from build123d import *

# Parameters (mm, degrees)
SKETCH_1_W            = 80
SKETCH_1_H            = 35
SKETCH_1_R            = 1.5
EXTRUDE_1_DEPTH       = 1.5
EXTRUDE_START         = 7
EXTRUDE_2_OUTLINE_W   = 71
EXTRUDE_2_OUTLINE_H   = 6
EXTRUDE_2_OUTLINE_H_2 = 2
EXTRUDE_2_DEPTH       = 22.5
EXTRUDE_2_2_OUTLINE_W = 44.5
EXTRUDE_2_2_OUTLINE_H = 10
EXTRUDE_2_2_DEPTH     = 3.5


# Read off the part's stored shape, not the designer's step: Бобышка-Вытянуть2
with BuildPart() as part:
    # Эскиз1 (on Top Plane) → Бобышка-Вытянуть1 (new body)
    with BuildSketch(Plane(origin=(0, 0, 0), x_dir=(1, 0, 0), z_dir=(0, 1, 0))):
        with Locations((40, -17.5)):
            Rectangle(SKETCH_1_W, SKETCH_1_H)
        with Locations(Location((2.5, -2, 0), (0, 0, 270))):
            Circle(SKETCH_1_R, mode=Mode.SUBTRACT)
        with Locations(Location((77.5, -2, 0), (0, 0, 90))):
            Circle(SKETCH_1_R, mode=Mode.SUBTRACT)
        with Locations(Location((77.5, -33, 0), (0, 0, 270))):
            Circle(SKETCH_1_R, mode=Mode.SUBTRACT)
        with Locations(Location((2.5, -33, 0), (0, 0, 90))):
            Circle(SKETCH_1_R, mode=Mode.SUBTRACT)
    extrude(amount=EXTRUDE_1_DEPTH)

    # Бобышка-Вытянуть2 outline → Бобышка-Вытянуть2 (add)
    with BuildSketch(Plane.XY.offset(EXTRUDE_START)):
        with Locations((40, 4.5)):
            Rectangle(EXTRUDE_2_OUTLINE_W, EXTRUDE_2_OUTLINE_H)
        with Locations((40, -1)):
            Rectangle(EXTRUDE_2_OUTLINE_W, EXTRUDE_2_OUTLINE_H_2)
    extrude(amount=EXTRUDE_2_DEPTH)

    # Extrude 2 2 outline → Extrude 2 2 (add)
    with BuildSketch(Plane.XY):
        with Locations((27.75, -5)):
            Rectangle(EXTRUDE_2_2_OUTLINE_W, EXTRUDE_2_2_OUTLINE_H)
    extrude(amount=EXTRUDE_2_2_DEPTH)


solid = part.part
Verification items for the finished model (mm, model axes). A direction names the side the tool comes from. Give positions to 0.01 mm unless a question says otherwise; leave off trailing zeros. Order: outer loops, then holes, each group sorted by start corner. A loop starts at its lowest first (then second) coordinate and runs counter-clockwise, first axis right, second up. Notation, with made-up numbers: (72.25, 20.25) -> (108.25, 20.25) arc R20 ccw to (108.25, 26.25) -> close; hole circle Ø6 at (9, -31.5). An arc over 180 degrees is marked (long way). Answer as CSV lines item,"result".
Q1. Sectioned sample at D-D on z = 15. Record the cut outline in (x, y), plus the area to 3 significant figures.
Solutions:
outline,"(0, 0) -> (4.5, 0) -> (4.5, -2) -> (75.5, -2) -> (75.5, 0) -> (80, 0) -> (80, 1.5) -> (75.5, 1.5) -> (75.5, 7.5) -> (4.5, 7.5) -> (4.5, 1.5) -> (0, 1.5) -> close"
area,"688 mm²"
Q2. Sectioned sample at C-C on x = 77.5. Record the cut outline in (y, z), plus the area to 3 significant figures.
Solutions:
outline,"(0, 0) -> (1.5, 0) -> (1.5, 0.5) -> (0, 0.5) -> close; (0, 3.5) -> (1.5, 3.5) -> (1.5, 31.5) -> (0, 31.5) -> close; (0, 34.5) -> (1.5, 34.5) -> (1.5, 35) -> (0, 35) -> close"
area,"43.5 mm²"
Q3. Sectioned sample at A-A on y = -1. Record the cut outline in (x, z), plus the area to 3 significant figures.
Solutions:
outline,"(4.5, 7) -> (75.5, 7) -> (75.5, 29.5) -> (4.5, 29.5) -> close; (5.5, 0) -> (50, 0) -> (50, 3.5) -> (5.5, 3.5) -> close"
area,"1,750 mm²"
Q4. Depth check by flat-ended pin: pin 1 (12 mm diameter, centred on x = 30, z = 15.5, fed in from -Y); pin 2 (3 mm diameter, centred on y = 3.5, z = 17, fed in from +X); pin 3 (1.8 mm diameter, centred on x = 2.5, z = 33, fed in from -Y); pin 4 (3 mm diameter, centred on y = -5.5, z = 2.5, fed in from +X). Enter the tip coordinate at first touch or a pass-through.
Solutions:
pin 1,"stops at y = -2"
pin 2,"stops at x = 75.5"
pin 3,"passes through"
pin 4,"stops at x = 50"
Q5. Sectioned sample at B-B on z = 2. Record the cut outline in (x, y), plus the area to 3 significant figures.
Solutions:
outline,"(0, 0) -> (1, 0) -> (1, 1.5) -> (0, 1.5) -> close; (4, 0) -> (5.5, 0) -> (5.5, -10) -> (50, -10) -> (50, 0) -> (76, 0) -> (76, 1.5) -> (4, 1.5) -> close; (79, 0) -> (80, 0) -> (80, 1.5) -> (79, 1.5) -> close"
area,"556 mm²"
Q6. Scan lines: probe 1 along X at (y, z) = (0.9, 2); probe 2 along Z at (x, y) = (77.5, 0.3); probe 3 along X at (y, z) = (2.75, 16.5). Record each from-to range of solid material in increasing order.
Solutions:
probe 1,"x = 0 to 1, 4 to 76, 79 to 80"
probe 2,"z = 0 to 0.5, 3.5 to 31.5, 34.5 to 35"
probe 3,"x = 4.5 to 75.5"
Q7. Access from +Z, -Z, +X, -X, +Y, -Y to the whole of each face (thin tool, end or side, straight path). Record for faces 1 (the flat face through (50, -5, 2)), 2 (the flat face through (5.5, -5, 2)), 3 (the flat face through (75.5, 4, 18)).
Solutions:
face 1,"-Z, +X, -Y"
face 2,"-Z, -X, -Y"
face 3,"+Z, -Z, +X, +Y"
Q8. Release check for a two-part mould opening along Z. For faces 4 (the flat face through (40, 0, 30)), 5 (the flat face through (39, 1, 35)), 6 (the flat face through (4.5, 4, 18)) record: +Z half, -Z half, draft (parallel to the pull), parting line (faces both ways), or undercut.
Solutions:
face 4,"undercut"
face 5,"+Z half"
face 6,"draft"
